Study the drawing (mm; zero at the part's minimum x, y, z) and answer. Coordinates: 2 decimals unless noted, no trailing zeros. Order: outer loops, then holes, each group sorted by start corner. A loop starts at its lowest first (then second) coordinate and runs counter-clockwise, first axis right, second up. Notation, with made-up numbers: (43.5, 22.25) -> (87.5, 22.25) arc R35 ccw to (87.5, 56.25) -> close; hole circle Ø6 at (-36, -13). An arc over 180 degrees is marked (long way). Answer in a Markdown table with one row per item. Add a question column.
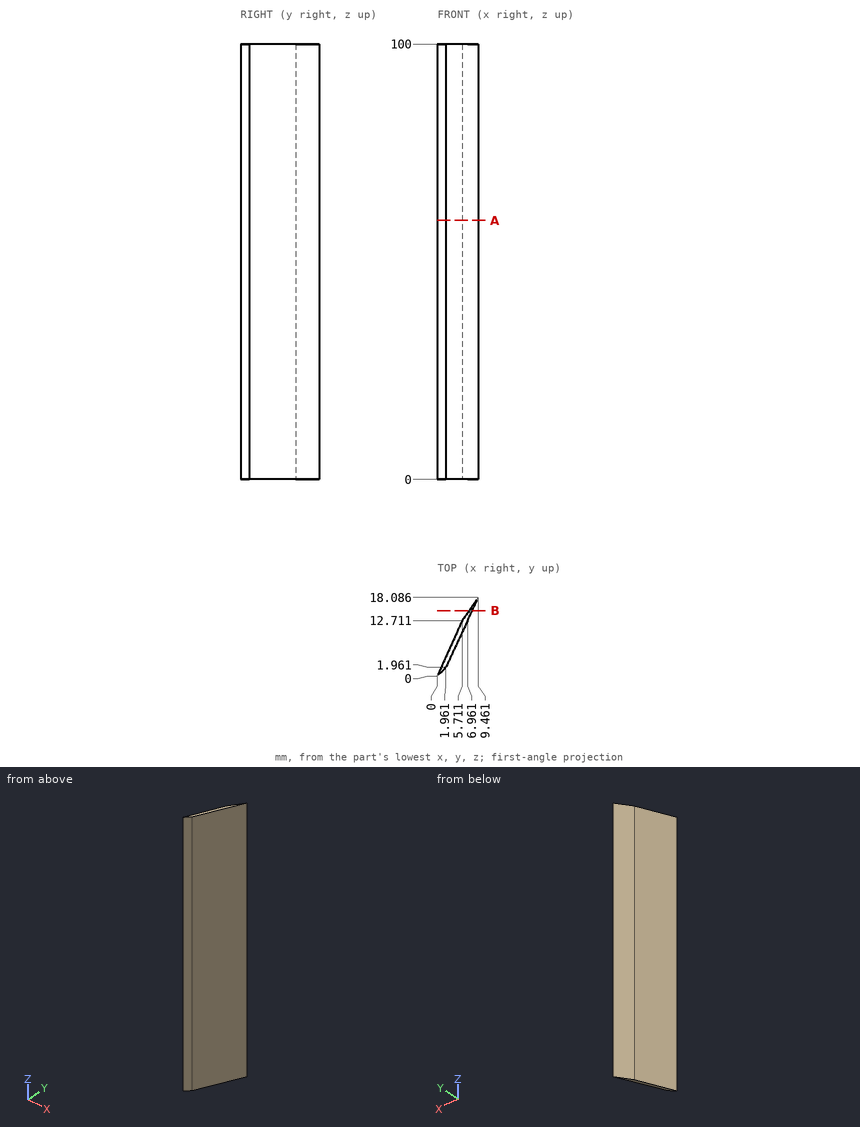
Q1. Given pin 1 (3 mm diameter, centred on y = 8.5, z = 55, fed in from +X); pin 2 (1.5 mm diameter, centred on y = 4, z = 19.5, fed in from +X); pin 3 (6 mm diameter, centred on y = 7.5, z = 64.5, fed in from -X), each flat-ended and moving along its own axis, determine where each tip first touches the part or whether it passes through.
Q2. Straight lines are drawn through the part: line 1 (X direction, y = 10.25, z = 12) (1 decimal); line 2 (Y direction, x = 6.75, z = 39) (1 decimal); line 3 (X direction, y = 2.5, z = 60.5). For each, find the intervals that lie inside material, in ascending order.
Q3. A cutting plane is placed at A-A (z = 59.5). Determine the outline of the cut face in (x, y).
Q4. A cutting plane is placed at B-B (y = 15). Determine the outline of the cut face in (x, z) (1 decimal).
Returned:
| question | item | result |
|---|---|---|
| 1 | pin 1 | stops at x = 5.7 |
| 1 | pin 2 | stops at x = 3.26 |
| 1 | pin 3 | stops at x = 2.02 |
| 2 | line 1 | x = 4.6 to 5.8 |
| 2 | line 2 | y = 12.3 to 14.2 |
| 2 | line 3 | x = 1.12 to 2.21 |
| 3 | outline | (0, 0) -> (1.96, 1.96) -> (9.46, 18.09) -> (5.71, 12.71) -> close |
| 4 | outline | (7.3, 0) -> (8, 0) -> (8, 100) -> (7.3, 100) -> close |
